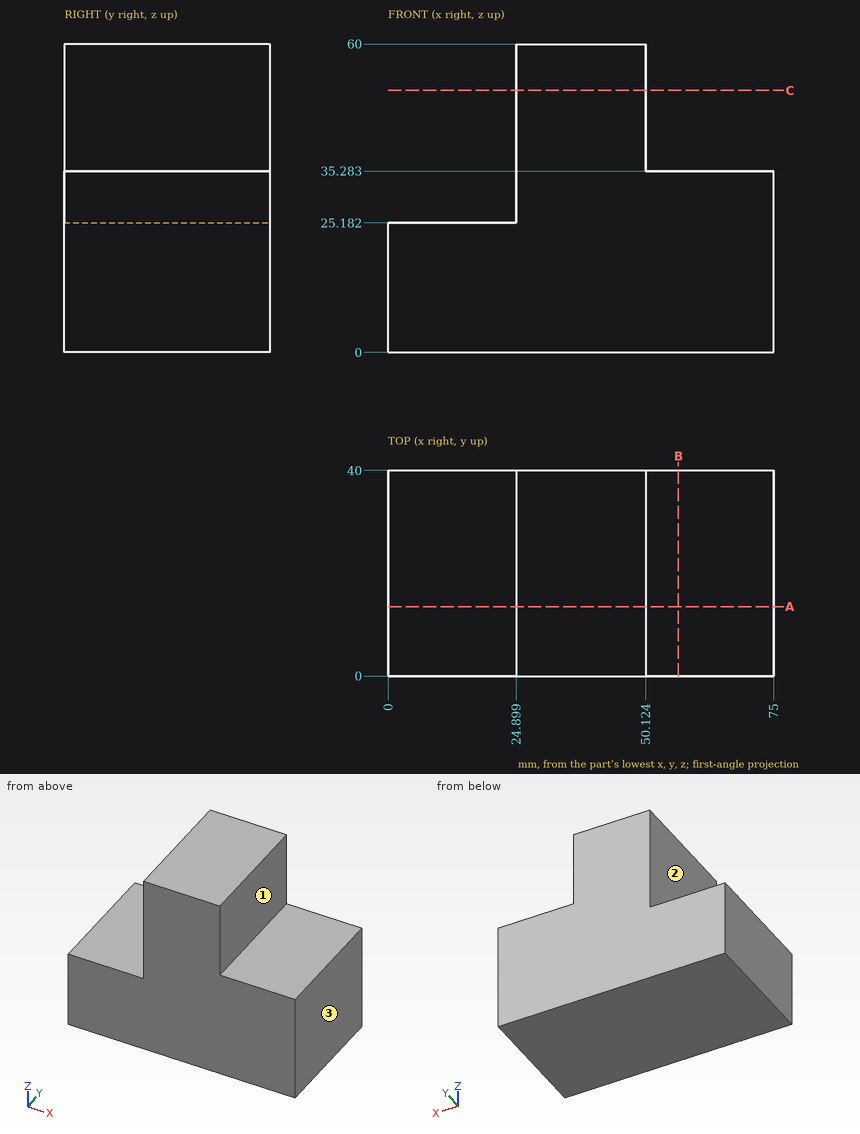
For this review, use the dimensioned drawing (mm, ordinates from the lowest corner) and the shaded views. A direction names the side the tool comes from. Give positions to 0.01 mm unless a question says otherwise; leave off trailing zeros. Order: outer loops, then holes, each group sorted by start corner. A loop starts at its lowest first (then second) coordinate and runs counter-clockwise, first axis right, second up. Notation, with made-up numbers: (-17.5, 88) - (14.5, 88) arc R25 cw to (14.5, 119) - close; hole circle Ø6 at (16, -9). An arc over 180 degrees is marked (long way). Write item = value, one per line. Start each with the question number.
Q1. To check wall thickness, follow L1, parallel to X at y = 17, z = 30.5; L2, parallel to X at y = 20, z = 41; L3, parallel to Z at x = 54, y = 30.5. State the ranges of each line that lie inside material, in increasing order. Write a range as from..to.
Q2. Clearance check with flat-ended pins moving along their axes: pin 1 Ø12.5 at (x, y) = (67, 21.5) entering from +Z; pin 2 Ø7.5 at (y, z) = (22.5, 50.5) entering from +X; pin 3 Ø7.5 at (x, y) = (8, 13.5) entering from +Z. State where each tip first meets the part, or that it passes through.
Q3. We need section A-A on y = 13.5. State the section outline as (x, z) points.
Q4. We need section B-B on x = 56.5. State the section outline as (y, z) points.
Q5. Tool access review of the marked faces 1, 2 and 3: name each direction out of +Z, -Z, +X, -X, +Y, -Y from which nothing blocks a thin tool from reaching the whole face with its end or side.
Q6. We need section C-C on z = 51. State the section outline as (x, y) points.
Working result:
q1.L1 = 24.9..75
q1.L2 = 24.9..50.12
q1.L3 = 0..35.28
q2.pin_1 = 35.28
q2.pin_2 = 50.12
q2.pin_3 = 25.18
q3.outline = (0, 0) - (75, 0) - (75, 35.28) - (50.12, 35.28) - (50.12, 60) - (24.9, 60) - (24.9, 25.18) - (0, 25.18) - close
q4.outline = (0, 0) - (40, 0) - (40, 35.28) - (0, 35.28) - close
q5.face_1 = +Z, +X, +Y, -Y
q5.face_2 = +Z, -X, +Y, -Y
q5.face_3 = +Z, -Z, +X, +Y, -Y
q6.outline = (24.9, 0) - (50.12, 0) - (50.12, 40) - (24.9, 40) - close
